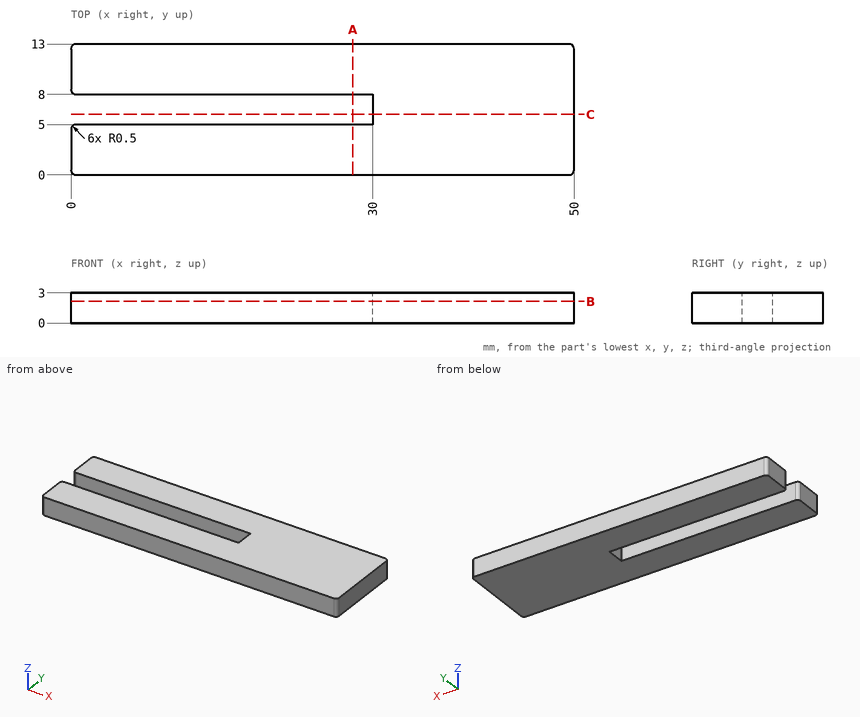
Design review of the part shown in the three views and the two pictorial views. Dimensions are in mm from the part's minimum x, y and z. Give positions to 0.01 mm unless a question says otherwise; leave off trailing zeros. Loops run counter-clockwise (first coordinate to the right, second up) from the corner with the lowest first, then second, coordinate; pieces in that order, holes last. Notation, with made-up numbers: M -19.5,-2.75 L -13.5,-2.75 A17 ccw -13.5,28.25 Z; hole C -15.75,35 d3. An arc over 180 degrees is marked long. Answer as a JSON object with one key per item and string values. Group by question number.
Q1. Add section C-C on y = 6. Give the boundary of the cut face in (x, z), and give its area (3 significant figures).
Q2. Add section B-B on z = 2.15. Give the boundary of the cut face in (x, y).
Q3. For probe 1 along Y at (x, z) = (3.5, 1.55); probe 2 along X at (y, z) = (5.25, 1.85), list the stretches that pass through material, from the lowest coordinate up. Write a range as [from, to].
Q4. Add section A-A on x = 28. Give the boundary of the cut face in (y, z), and give its area (3 significant figures).
Checked values:
{
 "1": {"outline": "M 30,0 L 50,0 L 50,3 L 30,3 Z", "area": "60.0 mm²"},
 "2": {"outline": "M 0,0.5 A0.5 ccw 0.5,0 L 49.5,0 A0.5 ccw 50,0.5 L 50,12.5 A0.5 ccw 49.5,13 L 0.5,13 A0.5 ccw 0,12.5 L 0,8.5 A0.5 ccw 0.5,8 L 30,8 L 30,5 L 0.5,5 A0.5 ccw 0,4.5 Z"},
 "3": {"probe 1": "[0, 5], [8, 13]", "probe 2": "[30, 50]"},
 "4": {"outline": "M 0,0 L 5,0 L 5,3 L 0,3 Z; M 8,0 L 13,0 L 13,3 L 8,3 Z", "area": "30.0 mm²"}
}
